```python
from build123d import *

# Parameters (mm, degrees)
F0_W     = 203.2
F0_H     = 127
F1_DEPTH = 127
F3_DEPTH = 76.2
F4_SIZE2 = 101.6
F4_SIZE  = 76.2
F5_R     = 5.08
F6_R     = 15.24
F7_DEPTH = 50.8
F8_R     = 19.05
F9_DEPTH = 127


with BuildPart() as f1:
    # F0 (on Front) → F1 (new body)
    with BuildSketch(Plane.XZ):
        with Locations((0.1851254753, -0.3465637565)):
            Rectangle(F0_W, F0_H)
    extrude(amount=F1_DEPTH)

    # F2 (on face) → F3 (cut)
    with BuildSketch(Plane.XZ.offset(127)):
        Polygon((101.7851254753, 63.1534362435), (0, 63.1534362435), (0, 0), (-37.9148745247, 0), (-37.9148745247, -63.8465637565), (101.7851254753, -63.8465637565), align=None)
    extrude(amount=-F3_DEPTH, mode=Mode.SUBTRACT)

    # F4
    f4_edges = [f1.edges().sort_by_distance(p)[0] for p in [
        (101.785125, -25.4, 63.153436),
    ]]
    f4_side = f1.faces().sort_by_distance((-21.603245, -52.585928, 63.153436))[0]
    chamfer(f4_edges, length=F4_SIZE, length2=F4_SIZE2, reference=f4_side)

    # F5
    f5_edges = [f1.edges().sort_by_distance(p)[0] for p in [
        (-50.707437, -127, 63.153436),
        (0, -88.9, 63.153436),
        (0, -127, 31.576718),
        (-18.957437, -127, 0),
        (-37.914875, -127, -31.923282),
        (-37.914875, -50.8, -31.923282),
        (12.792563, -50.8, 63.153436),
        (0, -50.8, 31.576718),
        (-37.914875, 0, 63.153436),
        (-101.414875, -63.5, 63.153436),
        (-101.414875, -127, -0.346564),
        (-101.414875, 0, -0.346564),
        (-69.664875, -127, -63.846564),
        (-37.914875, -88.9, -63.846564),
        (101.785125, -25.4, -63.846564),
        (0.185125, 0, -63.846564),
        (-101.414875, -63.5, -63.846564),
        (31.935125, -50.8, -63.846564),
    ]]
    fillet(f5_edges, radius=F5_R)

    # F6 (on face) → F7 (cut, through all)
    with BuildSketch(Plane.XZ.offset(50.8)):
        with Locations((17.9651254753, -18.1265637565)):
            Circle(F6_R)
    extrude(amount=-F7_DEPTH, mode=Mode.SUBTRACT)

    # F8 (on face) → F9 (cut, through all)
    with BuildSketch(Plane.XY.offset(63.1534362435)):
        with Locations((-70.9348745247, -96.52)):
            Circle(F8_R)
    extrude(amount=-F9_DEPTH, mode=Mode.SUBTRACT)


solid = f1.part
```
Design review of the part built by this model. Coordinates are the model's own, in mm. A direction names the side the tool comes from. Coordinates: 2 decimals unless noted, no trailing zeros. Loops run counter-clockwise (first coordinate to the right, second up) from the corner with the lowest first, then second, coordinate; pieces in that order, holes last. Notation, with made-up numbers: (-32, 50) - (26, 50) arc R14 cw to (26, 71) - close; hole circle Ø4 at (-2.5, 48.25). An arc over 180 degrees is marked (long way). Use CSV: the item, a comma, the result in double quotes. Start each with the question number.
1) Wall thickness on L1, parallel to X at y = -96, z = -1; L2, parallel to X at y = -55.5, z = 47; L3, parallel to X at y = -96, z = 17: over which ranges is each line inside the solid? List them lowest first. Write a range as from..to.
2) For pin 1 Ø2 at (x, y) = (-13.5, -57.5) entering from -Z; pin 2 Ø2 at (y, z) = (-71, -30) entering from +X; pin 3 Ø3 at (x, y) = (33, -43.5) entering from +Z, all flat-tipped, find the tip position at first contact; note any pin that passes through.
3) Consider section D-D on z = 17.5. Write out the cut boundary in (x, y).
4) Tool access review of faces 4 (the cylindrical face through (17.067, -49.272, 61.705)), 5 (the flat face through (101.785, -25, -49)), 6 (the cylindrical face through (35.42, -49.35, -62.32)): name each direction out of +Z, -Z, +X, -X, +Y, -Y from which nothing blocks a thin tool from reaching the whole face with its end or side.
5) Consider section C-C on y = -96.52. Write out the cut boundary in (x, z), then the cut area to 3 significant figures.
6) The part is to be moulded in two halves that separate along Y. For faces 1 (the cylindrical face through (4.11, -1.45, -62.32)), 2 (the cylindrical face through (-73.41, -77.63, 0.54)), 3 (the flat face through (-101.415, -63, -1)), say which applies: +Y half, -Y half, draft (parallel to the pull), parting line (faces both ways), or undercut.
7) Consider section B-B on x = 11.5. Write out the cut boundary in (y, z).
8) Consider section A-A on z = -14. Write out the cut boundary in (x, y).
Geometry says:
1,L1,"-101.41..-89.98, -51.89..-37.91"
1,L2,"-101.41..0.01"
1,L3,"-101.41..-89.98, -51.89..0"
2,pin 1,"z = 0"
2,pin 2,"x = -37.91"
2,pin 3,"z = 55.27"
3,outline,"(-101.41, -121.92) arc R5.08 ccw to (-96.33, -127) - (-5.08, -127) arc R5.08 ccw to (0, -121.92) - (0, -55.88) arc R5.08 cw to (5.08, -50.8) - (59.83, -50.8) - (59.83, 0) - (-96.33, 0) arc R5.08 ccw to (-101.41, -5.08) - close; hole circle Ø38.1 at (-70.93, -96.52)"
4,face 4,"+Z, +X, -Y"
4,face 5,"+Z, -Z, +X, +Y, -Y"
4,face 6,"-Z, +X, -Y"
5,outline,"(-101.41, -58.77) arc R5.08 ccw to (-96.33, -63.85) - (-89.98, -63.85) - (-89.98, 63.15) - (-96.33, 63.15) arc R5.08 ccw to (-101.41, 58.07) - close; (-51.88, -63.85) - (-42.99, -63.85) arc R5.08 ccw to (-37.91, -58.77) - (-37.91, 0) - (0, 0) - (0, 58.07) arc R5.08 ccw to (-5.08, 63.15) - (-51.88, 63.15) - close"
5,area,"5,600 mm^2"
6,face 1,"+Y half"
6,face 2,"undercut"
6,face 3,"draft"
7,outline,"(-50.8, -58.77) arc R5.08 ccw to (-45.72, -63.85) - (-5.08, -63.85) arc R5.08 ccw to (0, -58.77) - (0, -31.93) - (-50.8, -31.93) - close; (-50.8, -4.33) - (0, -4.33) - (0, 58.07) arc R5.08 ccw to (-5.08, 63.15) - (-45.72, 63.15) arc R5.08 ccw to (-50.8, 58.07) - close"
8,outline,"(-101.41, -121.92) arc R5.08 ccw to (-96.33, -127) - (-42.99, -127) arc R5.08 ccw to (-37.91, -121.92) - (-37.91, -55.88) arc R5.08 cw to (-32.83, -50.8) - (3.29, -50.8) - (3.29, 0) - (-96.33, 0) arc R5.08 ccw to (-101.41, -5.08) - close; (32.64, -50.8) - (83.45, -50.8) - (83.45, 0) - (32.64, 0) - close; hole circle Ø38.1 at (-70.93, -96.52)"
